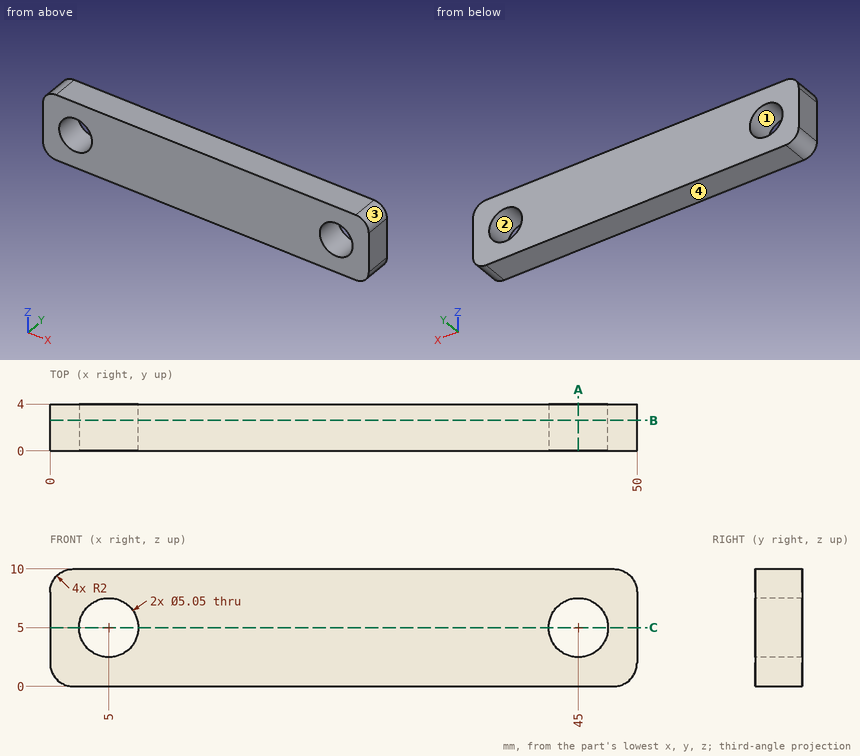
Print and shaded views of the part. All mm, measured from the part's lowest x, y and z. Coordinates: 2 decimals unless noted, no trailing zeros. Loops run counter-clockwise (first coordinate to the right, second up) from the corner with the lowest first, then second, coordinate; pieces in that order, holes last. Notation, with made-up numbers: (46.25, -12.5) - (64.25, -12.5) arc R26 cw to (64.25, 22.5) - close; hole circle Ø5 at (31.5, 51.5). An arc over 180 degrees is marked (long way). Write item = value, one per line. Start each with the question number.
Item 1: Cut at A-A, the plane x = 45. Give the cut face in (y, z) (3 decimals), and give its area (3 significant figures).
Item 2: Cut at C-C, the plane z = 5. Give the cut face in (x, y) (3 decimals).
Item 3: Flat gauge pin, fed straight in: pin 1 Ø4 at (x, z) = (45, 5) entering from +Y. Where does the tip first touch, or does it go through?
Item 4: Cut at B-B, the plane y = 2.6. Give the cut face in (x, z) (3 decimals), and give its area (3 significant figures).
Item 5: Wall check: L1, parallel to X at y = 1.1, z = 5 (3 decimals); L2, parallel to Z at x = 45, y = 0.95 (3 decimals); L3, parallel to X at y = 3.2, z = 6.25. Give the ranges that are in metal, low to high. Write a range as from..to.
Item 6: Mould opens along Z. For the marked faces 1, 2, 3 and 4 say: released by +Z, released by -Z, zero draft, split by the parting line, or undercut.
The answers:
q1.outline = (0, 0) - (4, 0) - (4, 2.475) - (0, 2.475) - close; (0, 7.525) - (4, 7.525) - (4, 10) - (0, 10) - close
q1.area = 19.8 mm2
q2.outline = (0, 0) - (2.475, 0) - (2.475, 4) - (0, 4) - close; (7.525, 0) - (42.475, 0) - (42.475, 4) - (7.525, 4) - close; (47.525, 0) - (50, 0) - (50, 4) - (47.525, 4) - close
q3.pin_1 = through
q4.outline = (0, 2) arc R2 ccw to (2, 0) - (48, 0) arc R2 ccw to (50, 2) - (50, 8) arc R2 ccw to (48, 10) - (2, 10) arc R2 ccw to (0, 8) - close; hole circle Ø5.05 at (5, 5); hole circle Ø5.05 at (45, 5)
q4.area = 457 mm2
q5.L1 = 0..2.475, 7.525..42.475, 47.525..50
q5.L2 = 0..2.475, 7.525..10
q5.L3 = 0..2.81, 7.19..42.81, 47.19..50
q6.face_1 = undercut
q6.face_2 = undercut
q6.face_3 = released by +Z
q6.face_4 = released by -Z
